Could you check a few things on this model? Use its own coordinates, in mm. A direction names the side the tool comes from. Give positions to 0.01 mm unless a question says otherwise; leave off trailing zeros. Loops run counter-clockwise (first coordinate to the right, second up) from the corner with the lowest first, then second, coordinate; pieces in that order, holes last.
1. Thinking about a two-plate mould opening in X: for faces 6 (the flat face through (1, 19.05, 0)), 7 (the flat face through (-38.1, 0, 0)), 8 (the cylindrical face through (-2.75, -12.4, 15.83)), 9 (the cylindrical face through (-7.559, -5.796, 22.181)), which applies, +X half, -X half, draft (parallel to the pull), parting line (faces both ways), or undercut?
2. For P1, Ø8, axis at y = 14, z = 17.5, coming from the +X side; P2, Ø2, axis at y = 11.5, z = 16, coming from the +X side; P3, Ø2, axis at x = 6, y = -3, coming from the -Z side; P4, Ø8, axis at x = 29.5, y = -0.5, coming from the +Z side, each with a flat end and sliding along its axis, tell me the tip position at first contact or that it passes through.
3. Imagine slicing it at C-C (z = 22). List the corners of the cut face in (x, y) for me (3 decimals).
4. I need wall thicknesses on line 1 along Y through (x, z) = (0, -15) (3 decimals); line 2 along Z through (x, y) = (26.5, -7); line 3 along X through (y, z) = (3, 6). Which ranges of each line are inside material? Lowest first, please.
5. Imagine slicing it at A-A (y = 0). List the corners of the cut face in (x, z) for me (3 decimals).
6. For faces 1 (the cylindrical face through (-15.12, -11.59, -15.74)), 2 (the cylindrical face through (-15.12, -11.59, 15.74)), 3 (the flat face through (27, 0, 6.35)), 4 (the flat face through (27, 0, -6.35)), 5 (the flat face through (5, 9, 19.05)), which set-ups out of +Z, -Z, +X, -X, +Y, -Y let a thin tool reach every point of the face, with its end or its side?
7. Imagine slicing it at D-D (y = 11). List the corners of the cut face in (x, z) for me.
```python
from build123d import *

# Parameters (mm, degrees)
F0_R          = 9.525
F1_DEPTH      = 6.35
F2_DEPTH      = 25.4
F2_DEPTH_BACK = 12.7
F3_R          = 19.05
F3_R_2        = 12.7
F3_R_3        = 9.525
F4_DEPTH      = 12.7
F5_DEPTH      = 6.35


with BuildPart() as f1:
    # F0 (on Top) → F1 (new body, symmetric)
    with BuildSketch(Plane.XY):
        with BuildLine():
            ThreePointArc((0, -19.05), (13.4703841816, -13.4703841816), (19.05, 0))
            ThreePointArc((19.05, 0), (13.4703841816, 13.4703841816), (0, 19.05))
            ThreePointArc((0, 19.05), (-19.05, 0), (0, -19.05))
        make_face()
        Circle(F0_R, mode=Mode.SUBTRACT)
        with BuildLine():
            ThreePointArc((0, 19.05), (13.4703841816, 13.4703841816), (19.05, 0))
            ThreePointArc((19.05, 0), (13.4703841816, -13.4703841816), (0, -19.05))
            Line((0, -19.05), (38.1, -19.05))
            Line((38.1, -19.05), (38.1, 19.05))
            Line((38.1, 19.05), (0, 19.05))
        make_face()
        with BuildLine():
            ThreePointArc((0, -19.05), (-19.05, 0), (0, 19.05))
            Line((0, 19.05), (-38.1, 19.05))
            Line((-38.1, 19.05), (-38.1, -19.05))
            Line((-38.1, -19.05), (0, -19.05))
        make_face()
    extrude(amount=F1_DEPTH, both=True)

    # F0 (on Top) → F2 (join, two sides)
    with BuildSketch(Plane.XY) as f2_sk:
        with BuildLine():
            ThreePointArc((0, -19.05), (13.4703841816, -13.4703841816), (19.05, 0))
            ThreePointArc((19.05, 0), (13.4703841816, 13.4703841816), (0, 19.05))
            ThreePointArc((0, 19.05), (-19.05, 0), (0, -19.05))
        make_face()
        Circle(F0_R, mode=Mode.SUBTRACT)
    extrude(amount=-F2_DEPTH)
    extrude(f2_sk.sketch, amount=F2_DEPTH_BACK)

    # F3 (on face) → F4 (join)
    with BuildSketch(Plane.XY.offset(12.7)):
        Circle(F3_R)
        Circle(F3_R_2, mode=Mode.SUBTRACT)
        Circle(F3_R_2)
        Circle(F3_R_3, mode=Mode.SUBTRACT)
    extrude(amount=F4_DEPTH)

    # F3 (on face) → F5 (cut)
    with BuildSketch(Plane.XY.offset(12.7)):
        Circle(F3_R_2)
        Circle(F3_R_3, mode=Mode.SUBTRACT)
    extrude(amount=F5_DEPTH, mode=Mode.SUBTRACT)


solid = f1.part
```
Derived:
1. face 6: draft
1. face 7: -X half
1. face 8: undercut
1. face 9: undercut
2. P1: stops at x = 16.21
2. P2: stops at x = 15.9
2. P3: passes through
2. P4: stops at z = 6.35
3. outline: circle Ø38.1 at (0, 0); hole circle Ø19.05 at (0, 0)
4. line 1: y = -19.05 to -9.525, 9.525 to 19.05
4. line 2: z = -6.35 to 6.35
4. line 3: x = -38.1 to -9.04, 9.04 to 38.1
5. outline: (-38.1, -6.35) - (-19.05, -6.35) - (-19.05, -25.4) - (-9.525, -25.4) - (-9.525, 12.7) - (-12.7, 12.7) - (-12.7, 19.05) - (-9.525, 19.05) - (-9.525, 25.4) - (-19.05, 25.4) - (-19.05, 6.35) - (-38.1, 6.35) - close; (9.525, -25.4) - (19.05, -25.4) - (19.05, -6.35) - (38.1, -6.35) - (38.1, 6.35) - (19.05, 6.35) - (19.05, 25.4) - (9.525, 25.4) - (9.525, 19.05) - (12.7, 19.05) - (12.7, 12.7) - (9.525, 12.7) - close
6. face 1: -Z
6. face 2: +Z
6. face 3: +Z, +X
6. face 4: -Z, +X
6. face 5: none
7. outline: (-38.1, -6.35) - (-15.55, -6.35) - (-15.55, -25.4) - (15.55, -25.4) - (15.55, -6.35) - (38.1, -6.35) - (38.1, 6.35) - (15.55, 6.35) - (15.55, 25.4) - (-15.55, 25.4) - (-15.55, 6.35) - (-38.1, 6.35) - close; hole (-6.35, 12.7) - (6.35, 12.7) - (6.35, 19.05) - (-6.35, 19.05) - close
